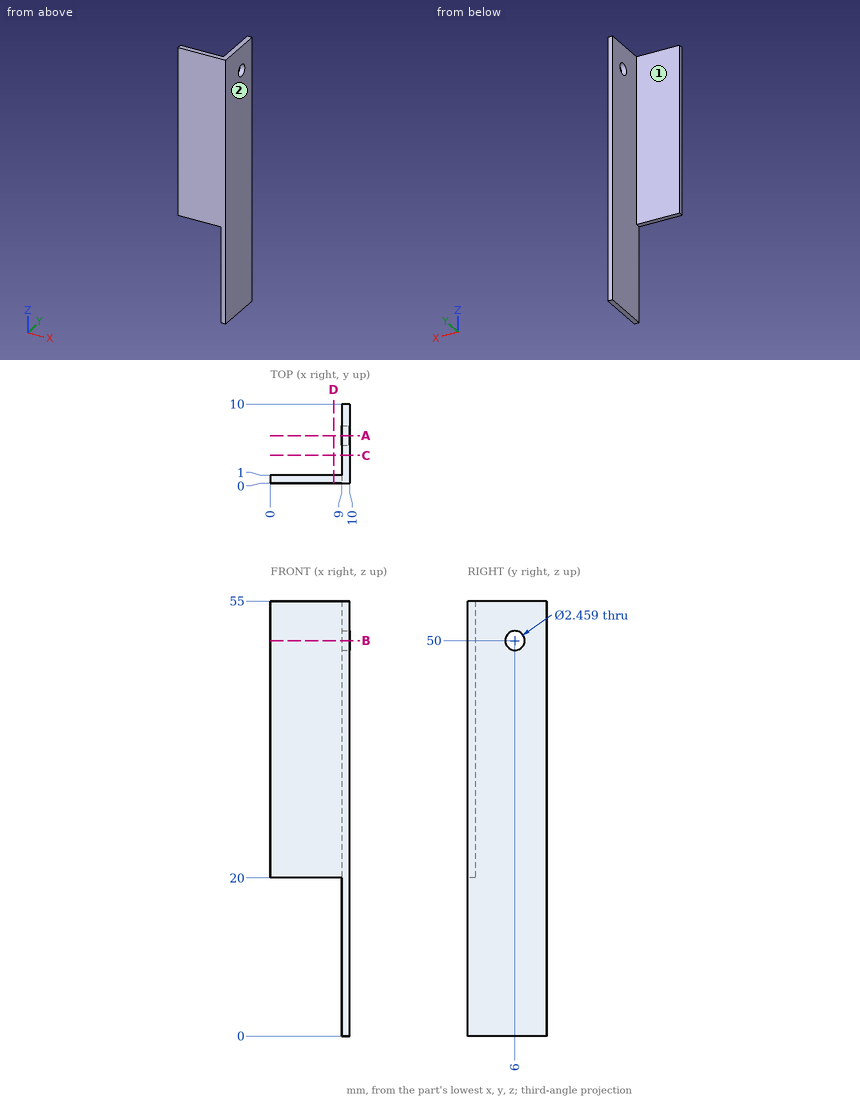
Job drawing, mm, ordinate dimensions from the low corner. One solid piece. A direction names the side the tool comes from. Give positions to 0.01 mm unless a question says otherwise; leave off trailing zeros. Order: outer loops, then holes, each group sorted by start corner. A loop starts at its lowest first (then second) coordinate and runs counter-clockwise, first axis right, second up. Notation, with made-up numbers: M 25,-34 L 70,-34 A17 cw 70,-27 Z; hole C 13,8 d9. An arc over 180 degrees is marked long. Put each result on its own line as item: value. Start each with the question number.
(1) Band-saw the part on A-A on y = 6. Give the cut face in (x, z), then the cut area to 3 significant figures.
(2) Band-saw the part on C-C on y = 3.5. Give the cut face in (x, z), then the cut area to 3 significant figures.
(3) Pin check, flat tips, straight feed: pin 1 Ø1.5 at (x, z) = (6.5, 14) entering from +Y; pin 2 Ø0.8 at (x, y) = (5.5, 0.5) entering from -Z; pin 3 Ø1 at (x, z) = (5, 29) entering from +Y; pin 4 Ø6 at (y, z) = (3.5, 14.5) entering from -X. Stop position of each tip, or through.
(4) Tool access for the marked faces 1 and 2: list every direction of +Z, -Z, +X, -X, +Y, -Y with a clear straight run to the whole face (end or side of a thin tool).
(5) Drill centre lines: L1, parallel to Z at x = 9.7, y = 6; L2, parallel to Y at x = 9.6, z = 50; L3, parallel to X at y = 5.5, z = 14.5. Where is each one in solid material? Low to high. Write a range as [from, to].
(6) Band-saw the part on B-B on z = 50. Give the cut face in (x, y).
(7) Band-saw the part on D-D on x = 8. Give the cut face in (y, z), then the cut area to 3 significant figures.
Results below:
1. outline: M 9,0 L 10,0 L 10,48.77 L 9,48.77 Z; M 9,51.23 L 10,51.23 L 10,55 L 9,55 Z
1. area: 52.5 mm2
2. outline: M 9,0 L 10,0 L 10,55 L 9,55 Z
2. area: 55.0 mm2
3. pin 1: passes through
3. pin 2: stops at z = 20
3. pin 3: stops at y = 1
3. pin 4: stops at x = 9
4. face 1: +Z, -Z, -X, +Y
4. face 2: +Z, -Z, +X, +Y, -Y
5. L1: z = [0, 48.77], [51.23, 55]
5. L2: y = [0, 4.77], [7.23, 10]
5. L3: x = [9, 10]
6. outline: M 0,0 L 10,0 L 10,4.77 L 9,4.77 L 9,1 L 0,1 Z; M 9,7.23 L 10,7.23 L 10,10 L 9,10 Z
7. outline: M 0,20 L 1,20 L 1,55 L 0,55 Z
7. area: 35.0 mm2
